Geometry: final body of the model. Coordinates: model frame, mm. A direction names the side the tool comes from. Give positions to 0.01 mm unless a question says otherwise; leave off trailing zeros. Write each loop counter-clockwise with the first axis right and the second up, starting at its lowest first coordinate (ties: lowest second). Pieces come first, ordered by that corner, then holes. Notation, with made-up numbers: M 63.25,24 L 87.25,24 A22 cw 87.25,40 Z; hole C -20,32.25 d6. An arc over 180 degrees is marked long. Answer as a JSON object with one key per item and string values.
from build123d import *

# Parameters (mm, degrees)
F0_R      = 250
F0_R_2    = 242.5
F6_DEPTH  = 25.4
F1_R      = 200
F1_R_2    = 192.5
F7_DEPTH  = 25.4
F2_R      = 150
F2_R_2    = 142.5
F8_DEPTH  = 25.4
F3_R      = 100
F3_R_2    = 92.5
F9_DEPTH  = 25.4
F4_R      = 50
F4_R_2    = 42.5
F10_DEPTH = 25.4
F5_R      = 25
F11_DEPTH = 25.4
F12_W     = 53.4157007933
F12_H     = 10.408022441
F12_W_2   = 10.0719733164
F12_H_2   = 50.3633767366
F12_W_3   = 52.6525899768
F12_H_3   = 9.6449414268
F12_H_4   = 41.9694781303
F12_H_5   = 22.8924434632
F12_W_4   = 30.523262918
F12_H_6   = 6.3797682524
F12_W_5   = 17.5508763641
F12_H_7   = 7.1428497322
F12_W_6   = 7.7827312052
F12_H_8   = 28.9970943704
F13_DEPTH = 25.4


with BuildPart() as f6:
    # F0 (on Top) → F6 (new body)
    with BuildSketch(Plane.XY):
        with Locations((-0.2296342573, -0.8695026627)):
            Circle(F0_R)
        with Locations((-1.2017333358, -0.1394655317)):
            Circle(F0_R_2, mode=Mode.SUBTRACT)
    extrude(amount=F6_DEPTH)



with BuildPart() as f7:
    # F1 (on Top) → F7 (new body)
    with BuildSketch(Plane.XY):
        with Locations((-0.229648911, 0.6240262301)):
            Circle(F1_R)
        with Locations((-0.229648911, -0.9403247815)):
            Circle(F1_R_2, mode=Mode.SUBTRACT)
    extrude(amount=F7_DEPTH)


with BuildPart() as f8:
    # F2 (on Top) → F8 (new body)
    with BuildSketch(Plane.XY):
        with Locations((-0.0088901297, -1.2084672926)):
            Circle(F2_R)
        with Locations((-0.0048156621, 1.2250516324)):
            Circle(F2_R_2, mode=Mode.SUBTRACT)
    extrude(amount=F8_DEPTH)


with BuildPart() as f9:
    # F3 (on Top) → F9 (new body)
    with BuildSketch(Plane.XY):
        with Locations((-1.9242773997, -2.7173017152)):
            Circle(F3_R)
        with Locations((-1.5612963189, -3.2658300582)):
            Circle(F3_R_2, mode=Mode.SUBTRACT)
    extrude(amount=F9_DEPTH)


with BuildPart() as f10:
    # F4 (on Top) → F10 (new body)
    with BuildSketch(Plane.XY):
        with Locations((-3.2166936435, 2.6153912768)):
            Circle(F4_R)
        with Locations((-2.5570748915, 3.2750012369)):
            Circle(F4_R_2, mode=Mode.SUBTRACT)
    extrude(amount=F10_DEPTH)


with BuildPart() as f11:
    # F5 (on Top) → F11 (new body)
    with BuildSketch(Plane.XY):
        with Locations((2.1465087775, 5.5706012063)):
            Circle(F5_R)
    extrude(amount=F11_DEPTH)


with BuildPart() as f6_1:
    add(f6.part)

    add(f7.part)  # F13 merges F7

    add(f8.part)  # F13 merges F8

    add(f9.part)  # F13 merges F9

    add(f10.part)  # F13 merges F10

    add(f11.part)  # F13 merges F11
    # F12 (on face) → F13 (join)
    with BuildSketch(Plane.XY):
        with Locations((-222.6678654552, -5.2040112205)):
            Rectangle(F12_W, F12_H)
        with Locations((5.0359866582, -172.9443594813)):
            Rectangle(F12_W_2, F12_H_2)
        with Locations((121.1003102362, -4.8224707134)):
            Rectangle(F12_W_3, F12_H_3)
        with Locations((5.0359866582, 70.097066462)):
            Rectangle(F12_W_2, F12_H_4)
        with Locations((5.0359866582, 37.6661056653)):
            Rectangle(F12_W_2, F12_H_5)
        with Locations((-31.8975038826, 3.1898841262)):
            Rectangle(F12_W_4, F12_H_6)
        with Locations((34.8721230403, 3.5714248661)):
            Rectangle(F12_W_5, F12_H_7)
        with Locations((3.8913656026, -27.9588955455)):
            Rectangle(F12_W_6, F12_H_8)
    extrude(amount=F13_DEPTH)


solid = f6_1.part
1) Cut plane A-A on x = -131. Return loops of the section in (y, z), and give its area (3 significant figures).
Geometry check:
{"outline": "M -213.94,0 L -204.98,0 L -204.98,25.4 L -213.94,25.4 Z; M -150.7,0 L -142.2,0 L -142.2,25.4 L -150.7,25.4 Z; M -74.29,0 L -54.87,0 L -54.87,25.4 L -74.29,25.4 Z; M 57.32,0 L 71.88,0 L 71.88,25.4 L 57.32,25.4 Z; M 140.32,0 L 151.95,0 L 151.95,25.4 L 140.32,25.4 Z; M 204.7,0 L 212.2,0 L 212.2,25.4 L 204.7,25.4 Z", "area": "1,790 mm2"}
2) Cut plane B-B on y = 182.5. Return loops of the section in (x, z), and give its area (3 significant figures).
Geometry check:
{"outline": "M -170.16,0 L -160.73,0 L -160.73,25.4 L -170.16,25.4 Z; M -83.42,0 L -58.59,0 L -58.59,25.4 L -83.42,25.4 Z; M 58.13,0 L 82.96,0 L 82.96,25.4 L 58.13,25.4 Z; M 158.33,0 L 169.7,0 L 169.7,25.4 L 158.33,25.4 Z", "area": "1,790 mm2"}
3) Contact query for flat-ended pins moving along their axis: P1, Ø12.5, axis at x = -222, z = 17, coming from the -Y side; P2, Ø12.5, axis at y = 69, z = 10, coming from the +X side; P3, Ø14, axis at x = 33.5, z = 14.5, coming from the +Y side. Output: stop coordinate, or through.
Geometry check:
{"P1": "stops at y = -127.56", "P2": "stops at x = 241.54", "P3": "stops at y = 247.7"}
4) Cut plane D-D on z = 12. Give the number of separate pieces and of enclosed holes in the cut face, and give its area (3 significant figures).
Geometry check:
{"separate pieces": "1", "enclosed holes": "8", "area": "38,600 mm2"}
5) Set-up query: faces 4 (the flat face through (-34, 6.38, 13)), 5 (the flat face through (17, 0, 0)). Return all of +Z, -Z, +X, -X, +Y, -Y with unobstructed straight access to the full face (end or side cutting, diameter ignored); none if empty.
Geometry check:
{"face 4": "+Z, -Z", "face 5": "-Z, +X, -X, +Y, -Y"}
6) Cut plane C-C on x = 106. Return loops of the section in (y, z).
Geometry check:
{"outline": "M -227.18,0 L -217.66,0 L -217.66,25.4 L -227.18,25.4 Z; M -168.83,0 L -161.48,0 L -161.48,25.4 L -168.83,25.4 Z; M -107.33,0 L -94.01,0 L -94.01,25.4 L -107.33,25.4 Z; M -9.64,0 L 0,0 L 0,25.4 L -9.64,25.4 Z; M 96.46,0 L 104.91,0 L 104.91,25.4 L 96.46,25.4 Z; M 159.59,0 L 170.08,0 L 170.08,25.4 L 159.59,25.4 Z; M 217.38,0 L 225.44,0 L 225.44,25.4 L 217.38,25.4 Z"}
7) Pull-direction query (X, two-part tool) for faces 1 (the cylindrical face through (-54.425, -244.925, 12.522)), 2 (the flat face through (17, 0, 25.4)), 3 (the flat face through (120, 0, 13)); classes: pulls with the +X half, pulls with the -X half, needs draft (parallel to the pull), parting line crosses it, or undercut.
Geometry check:
{"face 1": "parting line crosses it", "face 2": "needs draft", "face 3": "undercut"}
8) Line query: line 1 (Y direction, x = 176.5, z = 15.5); line 2 (Y direction, x = -216, z = 5.75); line 3 (Y direction, x = -165.5, z = 22). Output: solid intervals per line, ascending. Write a range as from..to.
Geometry check:
{"line 1": "y = -177.69..-165.15, -93.01..-77.25, 75.37..94.25, 164.87..175.95", "line 2": "y = -127.14..-112.69, -10.41..0, 112.41..125.4", "line 3": "y = -188.45..-178.5, -112.01..-99.64, 97.76..113.25, 178.22..186.71"}
